from build123d import *

# Parameters (mm, degrees)
F0_R        = 2.5
F1_DEPTH    = 20
F2_DEPTH    = 18
F4_DEPTH    = 12.5
F5_R        = 2
F6_T1_DEPTH = 22.7492112937


# Not quite as in the source:
# - a fillet or chamfer that OpenCascade refuses, or shapes differently, is made with other operations: its cross-section is extruded or revolved along the edge and cut away or added


with BuildPart() as f1:
    # F0 (on Top) → F1 (new body)
    with BuildSketch(Plane.XY):
        Polygon((11, 8), (-11, 8), (-15, 0), (-11, -8), (11, -8), (15, 0), align=None)
        Circle(F0_R, mode=Mode.SUBTRACT)
    extrude(amount=F1_DEPTH)

    # F2 (add): a face of the model
    f2_faces = [f1.faces().sort_by_distance(p)[0] for p in [
        (0, 7.66, 20),
    ]]
    extrude(f2_faces, amount=F2_DEPTH)

    # F3 (on Front) → F4 (cut, symmetric)
    with BuildSketch(Plane.XZ):
        with BuildLine():
            Line((5, 38.0777472107), (-5, 38.0777472107))
            ThreePointArc((-5, 38.0777472107), (0, 20.5), (5, 38.0777472107))
        make_face()
    extrude(amount=F4_DEPTH, both=True, mode=Mode.SUBTRACT)

    # F5
    f5_edges = [f1.edges().sort_by_distance(p)[0] for p in [
        (11, -8, 19),
        (15, 0, 19),
        (11, 8, 19),
        (-11, -8, 19),
        (-15, 0, 19),
        (-11, 8, 19),
    ]]
    fillet(f5_edges, radius=F5_R)

    # F6: chamfer of 1.5 on 2 edges, made by hand

    # F6_s2 → F6_t1 (cut)
    with BuildSketch(Plane.XZ.offset(-11.3746056469)):
        with BuildLine():
            Line((-6.4721431849, 38.0562963897), (-6.1455853598, 37.1704776118))
            Line((-6.1455853598, 37.1704776118), (-6.1261127101, 37.1476562202))
            ThreePointArc((-6.1261127101, 37.1476562202), (-5.6470472065, 37.6020890449), (-5.107295987, 37.9747368421))
            Line((-5.107295987, 37.9747368421), (-5.123475383, 38.03))
            ThreePointArc((-5.123475383, 38.03), (-5.7978092839, 38.03), (-6.4721431849, 38.0862963897))
            Line((-6.4721431849, 38.0862963897), (-6.4721431849, 38.0562963897))
        make_face()
        with BuildLine():
            Line((6.4721431849, 38.0562963897), (6.1455853598, 37.1704776118))
            Line((6.1455853598, 37.1704776118), (6.1261127101, 37.1476562202))
            ThreePointArc((6.1261127101, 37.1476562202), (5.6470472065, 37.6020890449), (5.107295987, 37.9747368421))
            Line((5.107295987, 37.9747368421), (5.123475383, 38.03))
            ThreePointArc((5.123475383, 38.03), (5.7978092839, 38.03), (6.4721431849, 38.0862963897))
            Line((6.4721431849, 38.0862963897), (6.4721431849, 38.0562963897))
        make_face()
    extrude(amount=F6_T1_DEPTH, mode=Mode.SUBTRACT)


solid = f1.part
Read the model definition and answer for the solid it produces. Units are mm, in the model's axes. Coordinates: 2 decimals unless noted, no trailing zeros. Write each loop counter-clockwise with the first axis right and the second up, starting at its lowest first coordinate (ties: lowest second). Pieces come first, ordered by that corner, then holes. Notation, with made-up numbers: (39.5, 57) -> (95.5, 57) arc R23 cw to (95.5, 65) -> close; hole circle Ø4 at (79, 11). An arc over 180 degrees is marked (long way). Return JSON: item names as keys, results as strings.
(1) The part is cut by section A-A on y = 0. Give the vertices of the cut face in (x, z).
Answers below:
{"outline": "(-14.76, 0) -> (-2.5, 0) -> (-2.5, 20.83) arc R9.5 cw to (-6.17, 37.23) -> (-6.45, 38) -> (-14.76, 38) -> close; (2.5, 0) -> (14.76, 0) -> (14.76, 38) -> (6.45, 38) -> (6.17, 37.23) arc R9.5 cw to (2.5, 20.83) -> close"}
(2) Each of these flat-tipped pins is pushed along its axis until it touches: P1, Ø1, axis at x = 1.5, y = -4, coming from the +Z side; P2, Ø1.5, axis at x = -6.5, y = -3, coming from the -Z side; P3, Ø4, axis at y = -3.5, z = 18.5, coming from the +X side; P4, Ø5, axis at y = -5, z = 29, coming from the -X side. Where does it stop, or does it pass through?
Answers below:
{"P1": "z = 20.71", "P2": "z = 0", "P3": "x = 14.25", "P4": "x = -13.75"}
(3) Consider line 1 along X through (y, z) = (0, 4.75); line 2 along Y through (x, z) = (0, 8.25); line 3 along Z through (x, y) = (0, 4.25). Determine where each line is inside the solid, lowest interval first. Write a range as from..to.
Answers below:
{"line 1": "-14.76..-2.5, 2.5..14.76", "line 2": "-8..-2.5, 2.5..8", "line 3": "0..20.5"}
(4) For a pull along Z with two mould halves and no side action, classify faces 1 (the flat face through (-13, 4, 19)), 2 (the cylindrical face through (4.613, -0.112, 21.695)), 3 (the flat face through (10, 0, 38)) as pulls with the +Z half, pulls with the -Z half, needs draft (parallel to the pull), parting line crosses it, or undercut.
Answers below:
{"face 1": "needs draft", "face 2": "undercut", "face 3": "pulls with the +Z half"}
(5) The part is cut by section B-B on z = 30. Give the vertices of the cut face in (x, y), then the cut area to 3 significant figures.
Answers below:
{"outline": "(-14.55, -0.89) -> (-11.55, -6.89) arc R2 ccw to (-9.76, -8) -> (-9.5, -8) -> (-9.5, 8) -> (-9.76, 8) arc R2 ccw to (-11.55, 6.89) -> (-14.55, 0.89) arc R2 ccw to start; (9.5, -8) -> (9.76, -8) arc R2 ccw to (11.55, -6.89) -> (14.55, -0.89) arc R2 ccw to (14.55, 0.89) -> (11.55, 6.89) arc R2 ccw to (9.76, 8) -> (9.5, 8) -> close", "area": "111 mm^2"}
(6) The part is cut by section D-D on y = 5.5. Give the vertices of the cut face in (x, z).
Answers below:
{"outline": "(-12.25, 0) -> (12.25, 0) -> (12.25, 38) -> (6.45, 38) -> (6.17, 37.23) arc R9.5 cw (long way) to (-6.17, 37.23) -> (-6.45, 38) -> (-12.25, 38) -> close"}
(7) The part is cut by section C-C on x = 0. Give the vertices of the cut face in (y, z).
Answers below:
{"outline": "(-8, 0) -> (-2.5, 0) -> (-2.5, 20.5) -> (-8, 20.5) -> close; (2.5, 0) -> (8, 0) -> (8, 20.5) -> (2.5, 20.5) -> close"}
